Read the model definition and answer for the solid it produces. Units are mm, in the model's axes. A direction names the side the tool comes from. Coordinates: 2 decimals unless noted, no trailing zeros. Order: outer loops, then holes, each group sorted by start corner. A loop starts at its lowest first (then second) coordinate and runs counter-clockwise, first axis right, second up. Notation, with made-up numbers: (40, -14) -> (50, -14) arc R12 ccw to (50, -5) -> close; hole circle Ø2 at (50.25, 69). An arc over 180 degrees is marked (long way). Return JSON: item names as keys, results as strings. Group by question number.
```python
from build123d import *

# Parameters (mm, degrees)
SKETCH2_W           = 83
SKETCH2_H           = 80
BOSS_EXTRUDE1_DEPTH = 35
SKETCH3_W           = 23
SKETCH3_H           = 23
CUT_EXTRUDE1_DEPTH  = 20
CUT_EXTRUDE11_REACH = 98.881
SKETCH21_R          = 1.65
CUT_EXTRUDE3_REACH  = 69.433
SKETCH8_W           = 15
SKETCH8_H           = 29
SKETCH10_R          = 3.35
CUT_EXTRUDE4_DEPTH  = 12
SKETCH11_W          = 83
SKETCH11_H          = 35
BOSS_EXTRUDE2_DEPTH = 2.25
SKETCH24_W          = 58.39763532
SKETCH24_H          = 3
CUT_EXTRUDE13_DEPTH = 25
SKETCH25_W          = 30
SKETCH25_H          = 3.363441727
CUT_EXTRUDE14_DEPTH = 25
CUT_EXTRUDE15_REACH = 70.792
SKETCH28_W          = 4.5
SKETCH28_H          = 22.250000153
FILLET2_R           = 2
SKETCH29_R          = 2.6
CUT_EXTRUDE16_DEPTH = 8
SKETCH30_R          = 2.6
CUT_EXTRUDE17_DEPTH = 8
SKETCH32_W          = 83
SKETCH32_H          = 35
BOSS_EXTRUDE5_DEPTH = 10


with BuildPart() as part:
    # Sketch2 → Boss-Extrude1 (new body)
    with BuildSketch(Plane(origin=(0, 0, 0), x_dir=(1, 0, 0), z_dir=(0, 1, 0))):
        Rectangle(SKETCH2_W, SKETCH2_H)
    extrude(amount=BOSS_EXTRUDE1_DEPTH)

    # Sketch3 → Cut-Extrude1 (cut)
    with BuildSketch(Plane(origin=(0, 35, 0), x_dir=(1, 0, 0), z_dir=(0, 1, 0))):
        with Locations((28, -26.254632213)):
            Rectangle(SKETCH3_W, SKETCH3_H)
        with Locations((28, 28.5)):
            Rectangle(SKETCH3_W, SKETCH3_H)
    cut_extrude1 = extrude(amount=-CUT_EXTRUDE1_DEPTH, mode=Mode.SUBTRACT)

    # Sketch21 → Cut-Extrude11 (cut, up to next)
    with BuildSketch(Plane.ZY.offset(-39.5), mode=Mode.PRIVATE) as cut_extrude11_sk1:
        with Locations((-36.241596758, 29.796951458)):
            Circle(SKETCH21_R)
    cut_extrude11_tool1 = extrude(cut_extrude11_sk1.sketch, amount=-CUT_EXTRUDE11_REACH, mode=Mode.PRIVATE) & part.part
    # Sketch21 → Cut-Extrude11 (cut, up to next)
    with BuildSketch(Plane.ZY.offset(-39.5), mode=Mode.PRIVATE) as cut_extrude11_sk2:
        with Locations((-36.241596399, 20.666302449)):
            Circle(SKETCH21_R)
    cut_extrude11_tool2 = extrude(cut_extrude11_sk2.sketch, amount=-CUT_EXTRUDE11_REACH, mode=Mode.PRIVATE) & part.part
    # Sketch21 → Cut-Extrude11 (cut, up to next)
    with BuildSketch(Plane.ZY.offset(-39.5), mode=Mode.PRIVATE) as cut_extrude11_sk3:
        with Locations((-21.24159988, 29.796951458)):
            Circle(SKETCH21_R)
    cut_extrude11_tool3 = extrude(cut_extrude11_sk3.sketch, amount=-CUT_EXTRUDE11_REACH, mode=Mode.PRIVATE) & part.part
    # Sketch21 → Cut-Extrude11 (cut, up to next)
    with BuildSketch(Plane.ZY.offset(-39.5), mode=Mode.PRIVATE) as cut_extrude11_sk4:
        with Locations((-21.24159988, 20.666302449)):
            Circle(SKETCH21_R)
    cut_extrude11_tool4 = extrude(cut_extrude11_sk4.sketch, amount=-CUT_EXTRUDE11_REACH, mode=Mode.PRIVATE) & part.part
    # Sketch21 → Cut-Extrude11 (cut, up to next)
    with BuildSketch(Plane.ZY.offset(-39.5), mode=Mode.PRIVATE) as cut_extrude11_sk5:
        with Locations((18.771463682, 29.796951458)):
            Circle(SKETCH21_R)
    cut_extrude11_tool5 = extrude(cut_extrude11_sk5.sketch, amount=-CUT_EXTRUDE11_REACH, mode=Mode.PRIVATE) & part.part
    # Sketch21 → Cut-Extrude11 (cut, up to next)
    with BuildSketch(Plane.ZY.offset(-39.5), mode=Mode.PRIVATE) as cut_extrude11_sk6:
        with Locations((33.771463682, 29.796951458)):
            Circle(SKETCH21_R)
    cut_extrude11_tool6 = extrude(cut_extrude11_sk6.sketch, amount=-CUT_EXTRUDE11_REACH, mode=Mode.PRIVATE) & part.part
    # Sketch21 → Cut-Extrude11 (cut, up to next)
    with BuildSketch(Plane.ZY.offset(-39.5), mode=Mode.PRIVATE) as cut_extrude11_sk7:
        with Locations((33.771463682, 19.796951458)):
            Circle(SKETCH21_R)
    cut_extrude11_tool7 = extrude(cut_extrude11_sk7.sketch, amount=-CUT_EXTRUDE11_REACH, mode=Mode.PRIVATE) & part.part
    # Sketch21 → Cut-Extrude11 (cut, up to next)
    with BuildSketch(Plane.ZY.offset(-39.5), mode=Mode.PRIVATE) as cut_extrude11_sk8:
        with Locations((18.771463682, 20.666302449)):
            Circle(SKETCH21_R)
    cut_extrude11_tool8 = extrude(cut_extrude11_sk8.sketch, amount=-CUT_EXTRUDE11_REACH, mode=Mode.PRIVATE) & part.part
    cut_extrude11_1 = cut_extrude11_tool1.solids().sort_by_distance((39.5, 29.796951, -36.241597))[0]
    add(cut_extrude11_1, mode=Mode.SUBTRACT)
    cut_extrude11_2 = cut_extrude11_tool2.solids().sort_by_distance((39.5, 20.666302, -36.241596))[0]
    add(cut_extrude11_2, mode=Mode.SUBTRACT)
    cut_extrude11_3 = cut_extrude11_tool3.solids().sort_by_distance((39.5, 29.796951, -21.2416))[0]
    add(cut_extrude11_3, mode=Mode.SUBTRACT)
    cut_extrude11_4 = cut_extrude11_tool4.solids().sort_by_distance((39.5, 20.666302, -21.2416))[0]
    add(cut_extrude11_4, mode=Mode.SUBTRACT)
    cut_extrude11_5 = cut_extrude11_tool5.solids().sort_by_distance((39.5, 29.796951, 18.771464))[0]
    add(cut_extrude11_5, mode=Mode.SUBTRACT)
    cut_extrude11_6 = cut_extrude11_tool6.solids().sort_by_distance((39.5, 29.796951, 33.771464))[0]
    add(cut_extrude11_6, mode=Mode.SUBTRACT)
    cut_extrude11_7 = cut_extrude11_tool7.solids().sort_by_distance((39.5, 19.796951, 33.771464))[0]
    add(cut_extrude11_7, mode=Mode.SUBTRACT)
    cut_extrude11_8 = cut_extrude11_tool8.solids().sort_by_distance((39.5, 20.666302, 18.771464))[0]
    add(cut_extrude11_8, mode=Mode.SUBTRACT)
    cut_extrude11 = cut_extrude11_1 + cut_extrude11_2 + cut_extrude11_3 + cut_extrude11_4 + cut_extrude11_5 + cut_extrude11_6 + cut_extrude11_7 + cut_extrude11_8  # Cut-Extrude11 as one shape, for the pattern or mirror that repeats it

    # Sketch8 → Cut-Extrude3 (cut, up to next)
    with BuildSketch(Plane(origin=(0, 35, 0), x_dir=(1, 0, 0), z_dir=(0, 1, 0)), mode=Mode.PRIVATE) as cut_extrude3_sk1:
        with Locations((-7.5, -0.300000153)):
            Rectangle(SKETCH8_W, SKETCH8_H)
    cut_extrude3_tool1 = extrude(cut_extrude3_sk1.sketch, amount=-CUT_EXTRUDE3_REACH, mode=Mode.PRIVATE) & part.part
    # Sketch8 → Cut-Extrude3 (cut, up to next)
    with BuildSketch(Plane(origin=(0, 35, 0), x_dir=(1, 0, 0), z_dir=(0, 1, 0)), mode=Mode.PRIVATE) as cut_extrude3_sk2:
        with Locations((7.5, -0.300000153)):
            Rectangle(SKETCH8_W, SKETCH8_H)
    cut_extrude3_tool2 = extrude(cut_extrude3_sk2.sketch, amount=-CUT_EXTRUDE3_REACH, mode=Mode.PRIVATE) & part.part
    add(cut_extrude3_tool1.solids().sort_by_distance((-7.5, 35, 0.3))[0], mode=Mode.SUBTRACT)
    add(cut_extrude3_tool2.solids().sort_by_distance((7.5, 35, 0.3))[0], mode=Mode.SUBTRACT)

    # Sketch10 → Cut-Extrude4 (cut)
    with BuildSketch(Plane.ZY.offset(-15)):
        with Locations((8.800000153, 30)):
            Circle(SKETCH10_R)
        with Locations((8.800000153, 5)):
            Circle(SKETCH10_R)
        with Locations((-7.199999847, 5)):
            Circle(SKETCH10_R)
        with Locations((-7.199999847, 30)):
            Circle(SKETCH10_R)
    extrude(amount=-CUT_EXTRUDE4_DEPTH, mode=Mode.SUBTRACT)

    # Sketch11 → Boss-Extrude2 (add)
    with BuildSketch(Plane(origin=(0, 0, -40), x_dir=(-1, 0, 0), z_dir=(0, 0, -1))):
        with Locations((0, 17.5)):
            Rectangle(SKETCH11_W, SKETCH11_H)
    extrude(amount=BOSS_EXTRUDE2_DEPTH)

    # Mirror1: Cut-Extrude1, Cut-Extrude11 across plane
    add(cut_extrude1.mirror(Plane(origin=(0, 0, 0), x_dir=(0, 0, 1), z_dir=(1, 0, 0))), mode=Mode.SUBTRACT)
    add(cut_extrude11.mirror(Plane(origin=(0, 0, 0), x_dir=(0, 0, 1), z_dir=(1, 0, 0))), mode=Mode.SUBTRACT)

    # Sketch24 → Cut-Extrude13 (cut)
    with BuildSketch(Plane(origin=(0, 35, 0), x_dir=(1, 0, 0), z_dir=(0, 1, 0))):
        with Locations((0, 18.499999847)):
            Rectangle(SKETCH24_W, SKETCH24_H)
    extrude(amount=-CUT_EXTRUDE13_DEPTH, mode=Mode.SUBTRACT)

    # Sketch25 → Cut-Extrude14 (cut)
    with BuildSketch(Plane(origin=(0, 35, 0), x_dir=(1, 0, 0), z_dir=(0, 1, 0))):
        with Locations((0, 15.881720711)):
            Rectangle(SKETCH25_W, SKETCH25_H)
    extrude(amount=-CUT_EXTRUDE14_DEPTH, mode=Mode.SUBTRACT)

    # Cut-Extrude15: up to this face of the body (flat: up to its plane)
    cut_extrude15_end = Plane(part.part.faces().sort_by_distance((0, 10, -17.560159309))[0])
    # Sketch28 → Cut-Extrude15 (cut, up to the picked face)
    with BuildSketch(Plane(origin=(0, 35, 0), x_dir=(1, 0, 0), z_dir=(0, 1, 0)), mode=Mode.PRIVATE) as cut_extrude15_sk1:
        with Locations((-26.94881766, 31.124999923)):
            Rectangle(SKETCH28_W, SKETCH28_H)
    cut_extrude15_tool1 = split(extrude(cut_extrude15_sk1.sketch, amount=-CUT_EXTRUDE15_REACH, mode=Mode.PRIVATE), bisect_by=cut_extrude15_end, keep=Keep.BOTH, mode=Mode.PRIVATE)
    # Sketch28 → Cut-Extrude15 (cut, up to the picked face)
    with BuildSketch(Plane(origin=(0, 35, 0), x_dir=(1, 0, 0), z_dir=(0, 1, 0)), mode=Mode.PRIVATE) as cut_extrude15_sk2:
        with Locations((26.94881766, 31.124999923)):
            Rectangle(SKETCH28_W, SKETCH28_H)
    cut_extrude15_tool2 = split(extrude(cut_extrude15_sk2.sketch, amount=-CUT_EXTRUDE15_REACH, mode=Mode.PRIVATE), bisect_by=cut_extrude15_end, keep=Keep.BOTH, mode=Mode.PRIVATE)
    add(cut_extrude15_tool1.solids().sort_by(Axis((-26.948818, 35, -31.125), (0, -1, 0)))[0], mode=Mode.SUBTRACT)
    add(cut_extrude15_tool2.solids().sort_by(Axis((26.948818, 35, -31.125), (0, -1, 0)))[0], mode=Mode.SUBTRACT)

    # Fillet2
    fillet2_edges = [part.edges().sort_by_distance(p)[0] for p in [
        (-24.69881766, 12.5, -19.999999847),
        (24.69881766, 12.5, -19.999999847),
    ]]
    fillet(fillet2_edges, radius=FILLET2_R)

    # Sketch29 → Cut-Extrude16 (cut)
    with BuildSketch(Plane.XY.offset(-19.999999847)):
        with Locations((0, 29.5)):
            Circle(SKETCH29_R)
        with Locations((-7, 22.5)):
            Circle(SKETCH29_R)
        with Locations((7, 22.5)):
            Circle(SKETCH29_R)
        with Locations((0, 15.5)):
            Circle(SKETCH29_R)
    extrude(amount=-CUT_EXTRUDE16_DEPTH, mode=Mode.SUBTRACT)

    # Sketch30 → Cut-Extrude17 (cut)
    with BuildSketch(Plane(origin=(0, 0, -17), x_dir=(-1, 0, 0), z_dir=(0, 0, -1))):
        with Locations((-18.6, 22.5)):
            Circle(SKETCH30_R)
        with Locations((18.6, 22.5)):
            Circle(SKETCH30_R)
    extrude(amount=-CUT_EXTRUDE17_DEPTH, mode=Mode.SUBTRACT)

    # Sketch32 → Boss-Extrude5 (add)
    with BuildSketch(Plane.XY.offset(40)):
        with Locations((0, 17.5)):
            Rectangle(SKETCH32_W, SKETCH32_H)
    extrude(amount=BOSS_EXTRUDE5_DEPTH)


solid = part.part
```
1. Find section A-A on x = 11.5. Determine the outline of the cut face in (y, z).
2. Find section B-B on z = -12. Determine the outline of the cut face in (x, y), and give its area (3 significant figures).
3. Straight lines are drawn through the part: L1, parallel to X at y = 25.5, z = 26.5; L2, parallel to Y at x = 22.5, z = -7.2; L3, parallel to Z at x = 10, y = 21.5. For each, find the intervals that lie inside material, in ascending order.
4. Given pin 1 (2.5 mm diameter, centred on y = 29.8, z = -21.24, fed in from -X); pin 2 (1.5 mm diameter, centred on x = 31, z = 30.5, fed in from +Y), each flat-ended and moving along its own axis, determine where each tip first touches the part or whether it passes through.
5. For a pull along Z with two mould halves and no side action, classify faces 6 (the face through (-28, 25, 14.755)), 7 (the face through (-29.199, 14, -32)), 8 (the face through (-39.5, 25, 26)), 9 (the face through (1, 18, -42.25)) as released by +Z, released by -Z, zero draft, split by the parting line, or undercut.
6. Which of the six approach directions +Z, -Z, +X, -X, +Y, -Y give full straight-line access (tool end or side, diameter ignored) to faces 1 (the face through (0, 16, -28)), 2 (the face through (18, 0, 3)), 3 (the face through (-40.486, 30.293, 20.345)), 4 (the face through (-28, 15, 26)), 5 (the face through (40.486, 31.433, -21.456))?
7. Find section C-C on y = 5. Determine the outline of the cut face in (x, z).
8. Find section D-D on z = -1. Determine the outline of the cut face in (x, y).
Result:
{
 "1": {"outline": "(0, -42.25) -> (35, -42.25) -> (35, -20) -> (10, -20) -> (10, -14.2) -> (0, -14.2) -> close; (0, 14.8) -> (35, 14.8) -> (35, 50) -> (0, 50) -> close"},
 "2": {"outline": "(-41.5, 0) -> (-15, 0) -> (-15, 35) -> (-41.5, 35) -> close; (15, 0) -> (41.5, 0) -> (41.5, 35) -> (15, 35) -> close; hole circle Ø5.2 at (-18.6, 22.5); hole circle Ø5.2 at (18.6, 22.5)", "area": "1,810 mm^2"},
 "3": {"L1": "-41.5 to -39.5, -16.5 to 16.5, 39.5 to 41.5", "L2": "0 to 1.65, 8.35 to 26.65, 33.35 to 35", "L3": "-42.25 to -20, 14.8 to 50"},
 "4": {"pin 1": "x = -16.5", "pin 2": "y = 15"},
 "5": {"face 6": "undercut", "face 7": "zero draft", "face 8": "undercut", "face 9": "released by -Z"},
 "6": {"face 1": "none", "face 2": "+Z, -Z, +X, -X, -Y", "face 3": "-X", "face 4": "+Y", "face 5": "+X"},
 "7": {"outline": "(-41.5, -42.25) -> (41.5, -42.25) -> (41.5, 50) -> (-41.5, 50) -> close; hole (-15, -14.2) -> (15, -14.2) -> (15, -10.55) -> (27, -10.55) -> (27, -3.85) -> (15, -3.85) -> (15, 5.45) -> (27, 5.45) -> (27, 12.15) -> (15, 12.15) -> (15, 14.8) -> (-15, 14.8) -> close"},
 "8": {"outline": "(-41.5, 0) -> (-15, 0) -> (-15, 35) -> (-41.5, 35) -> close; (15, 0) -> (41.5, 0) -> (41.5, 35) -> (15, 35) -> close"}
}
